Work out the finished part from the listing and answer in its coordinate system (mm). Coordinates: 2 decimals unless noted, no trailing zeros. Order: outer loops, then holes, each group sorted by start corner. A loop starts at its lowest first (then second) coordinate and runs counter-clockwise, first axis right, second up. Notation, with made-up numbers: (18, -26.75) - (59, -26.75) arc R3 ccw to (59, -21.75) - close; hole circle Ø7 at (62.25, 35). An arc over 180 degrees is marked (long way). Answer as a JSON object with one key per item and string values. Group by question number.
1) Section C-C (x = 25) is taken. Give the vertices of the cut face in (y, z), plus the area to 3 significant figures.
2) Find the intervals of material crossed by line 1 along Z through (x, y) = (25, 0.45); line 2 along Z through (x, y) = (-20, 0.7); line 3 along Z through (x, y) = (24, 0.8), in increasing order.
3) Section D-D (z = -16) is taken. Give the vertices of the cut face in (x, y), plus the area to 3 significant figures.
4) The mould has two halves that part along X. Classify faces 1 (the face through (26.1, 0.8, 45)), 2 (the face through (28, 0.8, 45.5)), 3 (the face through (2, 1.6, -1)): released by +X, released by -X, zero draft, split by the parting line, or undercut.
5) Section B-B (z = 45) is taken. Give the vertices of the cut face in (x, y).
6) Section A-A (x = -20) is taken. Give the vertices of the cut face in (y, z).
Autodesk Fusion 360 part; units mm, degrees
sketch "Sketch1" plane through (0, 0, 0) normal (0, 1, 0) x (1, 0, 0)
  line L0 (30, -47.5) -> (-30, -47.5)
  line L1 (-30, -47.5) -> (-30, 47.5)
  line L2 (-30, 47.5) -> (30, 47.5)
  line L3 (30, 47.5) -> (30, -47.5)
  line L4 (30, -47.5) -> (-30, 47.5) construction
  line L5 (-30, -47.5) -> (30, 47.5) construction
  dimension "d1" = 60
  dimension "d2" = 95
extrude "Extrude1" add sketch "Sketch1" along normal blind 1.6
chamfer "Chamfer1" distance 4 angle 45 2 edges at (30, 0.8, 47.5) (30, 0.8, -47.5)
sketch "Sketch2" plane through (0, 1.6, 0) normal (0, 1, 0) x (-1, 0, 0)
  line L0 (-30, -43.5) -> (-26, -47.5)
  line L1 (-26, -47.5) -> (30, -47.5)
  line L2 (30, -47.5) -> (30, 47.5)
  line L3 (30, 47.5) -> (-26, 47.5)
  line L4 (-26, 47.5) -> (-30, 43.5)
  line L5 (-30, 43.5) -> (-30, -43.5)
  line L6 (30, 0) -> (-12.828, 0) construction
  line L7 (30, -47.5) -> (25, -47.5)
  line L8 (25, -47.5) -> (25, 47.5)
  line L9 (25, 47.5) -> (30, 47.5)
  line L10 (30, 47.5) -> (30, -47.5)
  dimension "d24" = 5
extrude "Extrude2" cut sketch "Sketch2" against normal through all contours L1 L2 L3 L7 L8 L9 L10
sketch "Sketch3" plane through (0, 1.6, 0) normal (0, 1, 0) x (-1, 0, 0)
  line L0 (25, 47.5) -> (-26, 47.5)
  line L1 (-26, 47.5) -> (-30, 43.5)
  line L2 (-30, 43.5) -> (-30, -43.5)
  line L3 (-30, -43.5) -> (-26, -47.5)
  line L4 (-26, -47.5) -> (25, -47.5)
  circle A0 centre (20, -45) radius 1.1
  line L5 (25, -47.5) -> (25, 47.5)
  dimension "d11" = 20
  dimension "d12" = 45
  dimension "d13" = 2.2
extrude "Extrude3" cut sketch "Sketch3" against normal through all contours A0
pattern_linear "R-Pattern1" count 2 spacing 45 along (1, 0, 0) count 2 spacing 90 along (0, 0, 1) of "Extrude3"
sketch "Sketch4" plane through (0, 1.6, 0) normal (0, 1, 0) x (-1, 0, 0)
  circle A0 centre (20, 45) radius 1.1
  circle A1 centre (20, -45) radius 1.1
  line L0 (25, 47.5) -> (-26, 47.5)
  line L1 (-26, 47.5) -> (-30, 43.5)
  line L2 (-30, 43.5) -> (-30, -43.5)
  line L3 (-30, -43.5) -> (-26, -47.5)
  line L4 (-26, -47.5) -> (25, -47.5)
  line L5 (20, -24) -> (20, 17) construction
  line L6 (0, 0) -> (36, 0) construction
  circle A2 centre (20, -16) radius 1.05
  circle A3 centre (20, 16) radius 1.05
  circle A4 centre (-25, 45) radius 1.1
  circle A5 centre (-25, -45) radius 1.1
  line L7 (25, -47.5) -> (25, 47.5)
  dimension "d19" = 32
  dimension "d20" = 16
  dimension "d21" = 20
  dimension "d22" = 2.1
extrude "Extrude4" cut sketch "Sketch4" against normal through all contours A2 | A3
Report:
{
 "1": {"outline": "(0, -47.5) - (1.6, -47.5) - (1.6, -46.1) - (0, -46.1) - close; (0, -43.9) - (1.6, -43.9) - (1.6, 43.9) - (0, 43.9) - close; (0, 46.1) - (1.6, 46.1) - (1.6, 47.5) - (0, 47.5) - close", "area": "145 mm²"},
 "2": {"line 1": "z = -47.5 to -46.1, -43.9 to 43.9, 46.1 to 47.5", "line 2": "z = -47.5 to -46.1, -43.9 to -17.05, -14.95 to 14.95, 17.05 to 43.9, 46.1 to 47.5", "line 3": "z = -47.5 to -45.46, -44.54 to 44.54, 45.46 to 47.5"},
 "3": {"outline": "(-25, 0) - (-21.05, 0) - (-21.05, 1.6) - (-25, 1.6) - close; (-18.95, 0) - (30, 0) - (30, 1.6) - (-18.95, 1.6) - close", "area": "84.6 mm²"},
 "4": {"face 1": "undercut", "face 2": "released by +X", "face 3": "zero draft"},
 "5": {"outline": "(-25, 0) - (-21.1, 0) - (-21.1, 1.6) - (-25, 1.6) - close; (-18.9, 0) - (23.9, 0) - (23.9, 1.6) - (-18.9, 1.6) - close; (26.1, 0) - (28.5, 0) - (28.5, 1.6) - (26.1, 1.6) - close"},
 "6": {"outline": "(0, -47.5) - (1.6, -47.5) - (1.6, -46.1) - (0, -46.1) - close; (0, -43.9) - (1.6, -43.9) - (1.6, -17.05) - (0, -17.05) - close; (0, -14.95) - (1.6, -14.95) - (1.6, 14.95) - (0, 14.95) - close; (0, 17.05) - (1.6, 17.05) - (1.6, 43.9) - (0, 43.9) - close; (0, 46.1) - (1.6, 46.1) - (1.6, 47.5) - (0, 47.5) - close"}
}
